from build123d import *

# Parameters (mm, degrees)
F0_W     = 300
F0_H     = 180
F1_DEPTH = 25
F2_R     = 10
F3_DEPTH = 25.001
F4_SIZE  = 5


with BuildPart() as f1:
    # F0 (on Top) → F1 (new body)
    with BuildSketch(Plane.XY):
        Rectangle(F0_W, F0_H)
    extrude(amount=F1_DEPTH)

    # F2 (on face) → F3 (cut, through all)
    with BuildSketch(Plane.XY.offset(25)):
        with Locations((0, 64.087388)):
            Circle(F2_R)
        with Locations((-125.502721, 64.087388)):
            Circle(F2_R)
        with Locations((-125.502721, -65.912612)):
            Circle(F2_R)
        with Locations((0, -65.912612)):
            Circle(F2_R)
        with Locations((124.497279, -65.912612)):
            Circle(F2_R)
        with Locations((124.497279, 64.087388)):
            Circle(F2_R)
    extrude(amount=-F3_DEPTH, mode=Mode.SUBTRACT)

    # F4
    f4_edges = [f1.edges().sort_by_distance(p)[0] for p in [
        (0, 90, 25),
        (150, 0, 25),
        (0, -90, 25),
        (-150, 0, 25),
        (0, -90, 0),
        (150, 0, 0),
        (0, 90, 0),
        (-150, 0, 0),
    ]]
    chamfer(f4_edges, length=F4_SIZE)


solid = f1.part
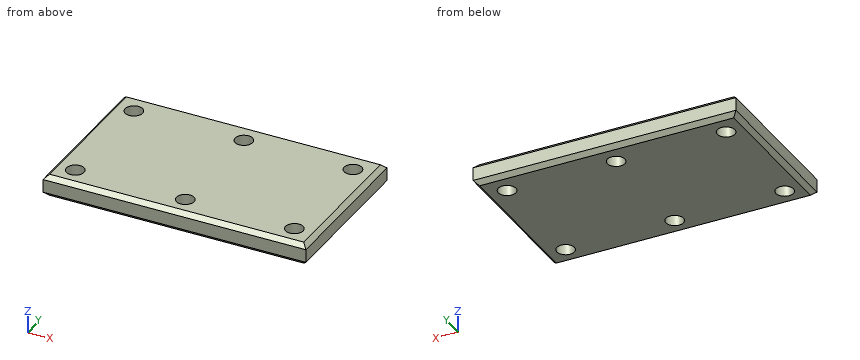
CAD build for the part. Positions are in the model's coordinates, mm. Round coordinates to 2 decimals unless told otherwise and drop trailing zeros. Write each loop counter-clockwise with the first axis right and the second up, starting at its lowest first coordinate (ties: lowest second). Pieces come first, ordered by that corner, then holes.
(1) Probe line 1 along Y through (x, z) = (0, 18.5); line 2 along X through (y, z) = (64, 5.75); line 3 along X through (y, z) = (-64.5, 9.5). List the from-to ranges inside material, lowest first.
(2) Drop a flat-ended pin along its axis: P1, Ø12, axis at x = 124.5, y = -65.91, coming from the +Z side. Give the stop position or say it passes through.
(3) Slice it at B-B, the plane z = 9.5. Write the cut outline in (x, y), and give its area (3 significant figures).
(4) Slice it at A-A, the plane x = 0. Write the cut outline in (y, z), and give its area (3 significant figures).
From the geometry:
1. line 1: y = -90 to -75.91, -55.91 to 54.09, 74.09 to 90
1. line 2: x = -150 to -135.5, -115.5 to -10, 10 to 114.5, 134.5 to 150
1. line 3: x = -150 to -135.4, -115.6 to -9.9, 9.9 to 114.6, 134.4 to 150
2. P1: passes through
3. outline: (-150, -90) - (150, -90) - (150, 90) - (-150, 90) - close; hole circle Ø20 at (-125.5, -65.91); hole circle Ø20 at (-125.5, 64.09); hole circle Ø20 at (0, -65.91); hole circle Ø20 at (0, 64.09); hole circle Ø20 at (124.5, -65.91); hole circle Ø20 at (124.5, 64.09)
3. area: 52,100 mm2
4. outline: (-90, 5) - (-85, 0) - (-75.91, 0) - (-75.91, 25) - (-85, 25) - (-90, 20) - close; (-55.91, 0) - (54.09, 0) - (54.09, 25) - (-55.91, 25) - close; (74.09, 0) - (85, 0) - (90, 5) - (90, 20) - (85, 25) - (74.09, 25) - close
4. area: 3,450 mm2
